Verification items for this drawing (mm, ordinates from the low corner). A direction names the side the tool comes from. Round coordinates to 2 decimals unless told otherwise and drop trailing zeros. Write each loop counter-clockwise with the first axis right and the second up, starting at its lowest first coordinate (ties: lowest second). Pieces come first, ordered by that corner, then holes.
Item 1: Scan lines: probe 1 along X at (y, z) = (162, 52) (3 decimals); probe 2 along Z at (x, y) = (378, 254) (3 decimals); probe 3 along Z at (x, y) = (127, 277). Record each from-to range of solid material in increasing order.
Item 2: Cross-section at B-B (z = 25.4). Enter the section's corners in (x, y) (3 decimals), then the cut area to 3 significant figures.
Item 3: Draft check along Y on the marked faces 4, 5 and 6. Enter one of: pulls with the +Y half, pulls with the -Y half, needs draft (parallel to the pull), parting line crosses it, or undercut.
Item 4: Cross-section at A-A (y = 254). Enter the section's corners in (x, z) (3 decimals), then the cut area to 3 significant figures.
Item 5: Cross-section at D-D (z = 142.5). Enter the section's corners in (x, y) (3 decimals).
Item 6: Depth check by flat-ended pin: P1, Ø17, axis at y = 254, z = 50.8, coming from the +X side (3 decimals); P2, Ø10, axis at x = 190, z = 15.5, coming from the -Y side; P3, Ø12, axis at y = 99.5, z = 83.5, coming from the +X side. Enter the tip coordinate at first touch or a pass-through.
Item 7: Cross-section at C-C (x = 127). Enter the section's corners in (y, z) (3 decimals), then the cut area to 3 significant figures.
Item 8: Access from +Z, -Z, +X, -X, +Y, -Y to the whole of each face (thin tool, end or side, straight path). Record for the marked faces 1, 2 and 3.
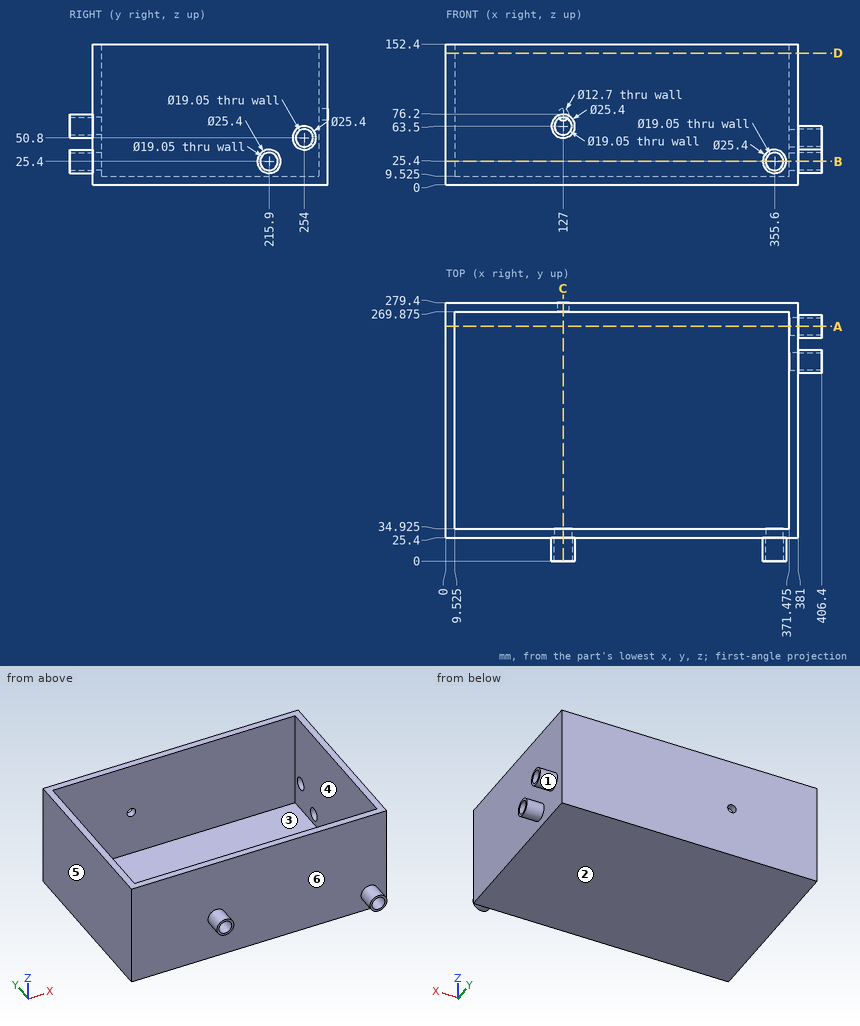
Resolved:
1. probe 1: x = 0 to 9.525, 371.475 to 381
1. probe 2: z = 0 to 41.275, 60.325 to 152.4
1. probe 3: z = 0 to 69.85, 82.55 to 152.4
2. outline: (0, 25.4) - (342.9, 25.4) - (342.9, 0) - (346.075, 0) - (346.075, 34.925) - (9.525, 34.925) - (9.525, 269.875) - (371.475, 269.875) - (371.475, 225.425) - (406.4, 225.425) - (406.4, 228.6) - (381, 228.6) - (381, 279.4) - (0, 279.4) - close; (365.125, 0) - (368.3, 0) - (368.3, 25.4) - (381, 25.4) - (381, 203.2) - (406.4, 203.2) - (406.4, 206.375) - (371.475, 206.375) - (371.475, 34.925) - (365.125, 34.925) - close
2. area: 11,700 mm2
3. face 4: undercut
3. face 5: needs draft
3. face 6: pulls with the -Y half
4. outline: (0, 0) - (381, 0) - (381, 38.1) - (406.4, 38.1) - (406.4, 41.275) - (371.475, 41.275) - (371.475, 9.525) - (9.525, 9.525) - (9.525, 152.4) - (0, 152.4) - close; (371.475, 60.325) - (406.4, 60.325) - (406.4, 63.5) - (381, 63.5) - (381, 152.4) - (371.475, 152.4) - close
4. area: 6,330 mm2
5. outline: (0, 25.4) - (381, 25.4) - (381, 279.4) - (0, 279.4) - close; hole (9.525, 34.925) - (371.475, 34.925) - (371.475, 269.875) - (9.525, 269.875) - close
6. P1: stops at x = 9.525
6. P2: stops at y = 25.4
6. P3: stops at x = 381
7. outline: (0, 50.8) - (25.4, 50.8) - (25.4, 0) - (279.4, 0) - (279.4, 69.85) - (269.875, 69.85) - (269.875, 9.525) - (34.925, 9.525) - (34.925, 53.975) - (0, 53.975) - close; (0, 73.025) - (34.925, 73.025) - (34.925, 152.4) - (25.4, 152.4) - (25.4, 76.2) - (0, 76.2) - close; (269.875, 82.55) - (279.4, 82.55) - (279.4, 152.4) - (269.875, 152.4) - close
7. area: 5,000 mm2
8. face 1: +X
8. face 2: -Z, +X, -X, +Y, -Y
8. face 3: +Z
